Can you work these out from the model? Positions are in its coordinate system, mm. A direction names the side the tool comes from. Coordinates: 2 decimals unless noted, no trailing zeros. Loops run counter-clockwise (first coordinate to the right, second up) from the corner with the lowest first, then second, coordinate; pieces in that order, holes last. Notation, with made-up numbers: (-6, 25) -> (45, 25) arc R15 ccw to (45, 48) -> close; hole circle Ø10 at (37, 38.25). An arc over 180 degrees is marked (long way). Use one line per item in the form item = value. Start each with the question number.
(1) Imagine slicing it at D-D (y = -18.5). List the corners of the cut face in (x, z) for me, plus the area to 3 significant figures.
(2) Imagine slicing it at B-B (y = 8). List the corners of the cut face in (x, z) for me, plus the area to 3 significant figures.
(3) Imagine slicing it at C-C (x = -15). List the corners of the cut face in (y, z) for me, plus the area to 3 significant figures.
(4) I'm going to push flat-ended pins straight in: pin 1 (1 mm diameter, centred on x = -68, y = -26, fed in from +Z); pin 2 (12.5 mm diameter, centred on x = -53, y = 5.5, fed in from +Z); pin 3 (15 mm diameter, centred on x = -56, z = 14, fed in from -Y). Where does each tip first touch, or does it pass through?
(5) On a 3-axis mill with a long thin cutter (end or side, diameter ignored), from which of +Z, -Z, +X, -X, +Y, -Y can I reach the whole of each face in a straight line? I mean faces 1 (the flat face through (-50, 29.259, -6)), 2 (the flat face through (-25.4, 4, 13)), 3 (the flat face through (-50, -8.841, -9)). Say none if no direction works.
(6) Imagine slicing it at A-A (z = 17). List the corners of the cut face in (x, y) for me.
(7) I need wall thicknesses on line 1 (Z direction, x = -40, y = -18); line 2 (Y direction, x = -88, z = 16); line 3 (X direction, y = 0.5, z = 6). Which ranges of each line are inside material? Lowest first, please. Write a range as [from, to].
(8) Thinking about a two-plate mould opening in X: for faces 4 (the flat face through (-50, -34.241, -31)), 5 (the flat face through (-76.2, 4, 13)), 6 (the flat face through (0, 4, -13)), which applies, released by +X, released by -X, zero draft, split by the parting line, or undercut?
```python
from build123d import *

# Parameters (mm, degrees)
F1_DEPTH = 101.6
F2_W     = 50.8
F2_H     = 38.1
F3_DEPTH = 25.4


with BuildPart() as f1:
    # F0 (on Right) → F1 (new body)
    with BuildSketch(Plane.YZ):
        Polygon((-34.241207, -18.016895), (-34.241207, -43.416895), (29.258793, -43.416895), (29.258793, 32.783105), (-8.841207, 32.783105), (-8.841207, -18.016895), align=None)
    extrude(amount=-F1_DEPTH)

    # F2 (on face) → F3 (cut)
    with BuildSketch(Plane.XZ.offset(8.841207)):
        with Locations((-50.8, 13.733105)):
            Rectangle(F2_W, F2_H)
    extrude(amount=-F3_DEPTH, mode=Mode.SUBTRACT)


solid = f1.part
```
Worked out:
q1.outline = (-101.6, -43.42) -> (0, -43.42) -> (0, -18.02) -> (-101.6, -18.02) -> close
q1.area = 2,580 mm2
q2.outline = (-101.6, -43.42) -> (0, -43.42) -> (0, 32.78) -> (-25.4, 32.78) -> (-25.4, -5.32) -> (-76.2, -5.32) -> (-76.2, 32.78) -> (-101.6, 32.78) -> close
q2.area = 5,810 mm2
q3.outline = (-34.24, -43.42) -> (29.26, -43.42) -> (29.26, 32.78) -> (-8.84, 32.78) -> (-8.84, -18.02) -> (-34.24, -18.02) -> close
q3.area = 3,550 mm2
q4.pin_1 = -18.02
q4.pin_2 = -5.32
q4.pin_3 = 16.56
q5.face_1 = +Z, -Z, +X, -X, +Y
q5.face_2 = +Z, -Y
q5.face_3 = +Z, +X, -X, -Y
q6.outline = (-101.6, -8.84) -> (-76.2, -8.84) -> (-76.2, 16.56) -> (-25.4, 16.56) -> (-25.4, -8.84) -> (0, -8.84) -> (0, 29.26) -> (-101.6, 29.26) -> close
q7.line_1 = [-43.42, -18.02]
q7.line_2 = [-8.84, 29.26]
q7.line_3 = [-101.6, -76.2], [-25.4, 0]
q8.face_4 = zero draft
q8.face_5 = undercut
q8.face_6 = released by +X
